from build123d import *

# Parameters (mm, degrees)
SKETCH2_W            = 100
SKETCH2_H            = 5.75
BOSS_EXTRUDE1_DEPTH  = 50
SKETCH4_R            = 11
CUT_EXTRUDE1_DEPTH   = 112.951161227
M3_CLEARANCE_HOLE2_D = 3.4
CUT_EXTRUDE3_DEPTH   = 5.75
FILLET1_R            = 25
FILLET2_R            = 10
M3_CLEARANCE_HOLE3_D = 3.4
SKETCH12_R           = 1
SKETCH12_W           = 24.5
SKETCH12_H           = 15
CUT_EXTRUDE4_DEPTH   = 5.75


with BuildPart() as part:
    # Sketch2 → Boss-Extrude1 (new body)
    with BuildSketch(Plane(origin=(0, 0, 0), x_dir=(1, 0, 0), z_dir=(0, 1, 0))):
        with Locations((-50, 2.875)):
            Rectangle(SKETCH2_W, SKETCH2_H)
    extrude(amount=BOSS_EXTRUDE1_DEPTH)

    # Sketch4 → Cut-Extrude1 (cut, through all)
    with BuildSketch(Plane.XY):
        with Locations((-25, 25)):
            Circle(SKETCH4_R)
    extrude(amount=-CUT_EXTRUDE1_DEPTH, mode=Mode.SUBTRACT)

    # M3 Clearance Hole2 (through all)
    with Locations(Plane.XY):
        with Locations((-35.606601718, 14.393398282), (-35.606601718, 35.606601718), (-14.393398282, 35.606601718), (-14.393398282, 14.393398282)):
            Hole(M3_CLEARANCE_HOLE2_D / 2)

    # Sketch9 → Cut-Extrude3 (cut)
    with BuildSketch(Plane.XY):
        with BuildLine():
            Line((-25, 50), (-100, 50))
            Line((-100, 50), (-100, 32.5))
            Line((-100, 32.5), (-48.848480035, 32.5))
            ThreePointArc((-48.848480035, 32.5), (-39.790199458, 45.155644371), (-25, 50))
        make_face()
        with BuildLine():
            Line((-25, 0), (-100, 0))
            Line((-100, 0), (-100, 17.5))
            Line((-100, 17.5), (-48.848480035, 17.5))
            ThreePointArc((-48.848480035, 17.5), (-39.790199458, 4.844355629), (-25, 0))
        make_face()
    extrude(amount=-CUT_EXTRUDE3_DEPTH, mode=Mode.SUBTRACT)

    # Fillet1
    fillet1_edges = [part.edges().sort_by_distance(p)[0] for p in [
        (0, 0, -2.875),
        (0, 50, -2.875),
    ]]
    fillet(fillet1_edges, radius=FILLET1_R - 0.0001)  # a hair under: the kernel refuses the full size

    # Fillet2
    fillet2_edges = [part.edges().sort_by_distance(p)[0] for p in [
        (-48.848480035, 32.5, -2.875),
        (-48.848480035, 17.5, -2.875),
    ]]
    fillet(fillet2_edges, radius=FILLET2_R)

    # M3 Clearance Hole3 (through all)
    with Locations(Plane.XY):
        with Locations((-94, 28.5), (-94, 21.5)):
            Hole(M3_CLEARANCE_HOLE3_D / 2)

    # Sketch12 → Cut-Extrude4 (cut)
    with BuildSketch(Plane.XY):
        with Locations((-70, 27.5)):
            Circle(SKETCH12_R)
        with Locations((-70, 22.5)):
            Circle(SKETCH12_R)
        with Locations((-87.75, 25)):
            Rectangle(SKETCH12_W, SKETCH12_H)
    extrude(amount=-CUT_EXTRUDE4_DEPTH, mode=Mode.SUBTRACT)


solid = part.part
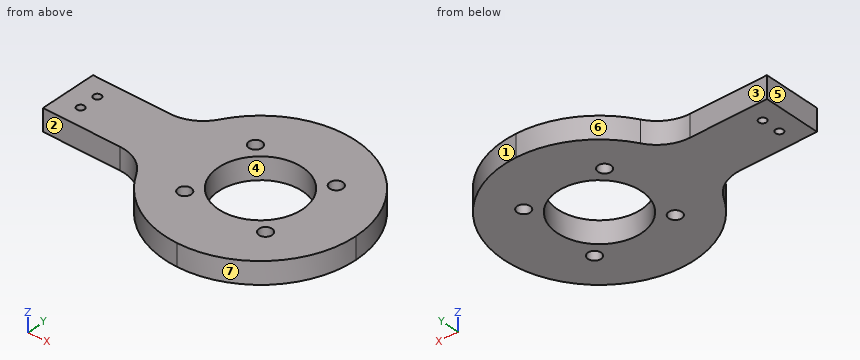
Work out the finished part from the listing and answer in its coordinate system (mm). Face numbers are marked on the shaded views. A direction names the side the tool comes from. Coordinates: 2 decimals unless noted, no trailing zeros. Loops run counter-clockwise (first coordinate to the right, second up) from the corner with the lowest first, then second, coordinate; pieces in that order, holes last. Notation, with made-up numbers: M 1,-10 L 23,-10 A29 cw 23,18 Z; hole C 44.5,62.5 d7. An arc over 180 degrees is marked long. Answer in a Markdown table with one row per item. Add a question column.
1. Consider L1, parallel to Y at x = -70, z = -2.25; L2, parallel to Y at x = -25, z = -4.2; L3, parallel to X at y = 37, z = -1.7. Determine where each line is inside the solid, lowest interval first.
2. The mould has two halves that part along Y. Classify the marked faces 4, 5, 6 and 7: pulls with the +Y half, pulls with the -Y half, needs draft (parallel to the pull), parting line crosses it, or undercut.
3. Find section A-A, the plane y = 22.5. Write down the section's boundary in (x, z), then the cut area to 3 significant figures.
4. Find section B-B, the plane x = -70. Write down the section's boundary in (y, z), then the cut area to 4 significant figures.
5. Find section C-C, the plane z = -4.5. State how many separate pieces and enclosed holes the cut face has, then the cut area to 3 significant figures.
6. Flat-ended cylindrical pins translate along their axes: P1, Ø2.5, axis at x = -35.61, y = 35.61, coming from the +Z side; P2, Ø2, axis at y = 13, z = -2.5, coming from the +X side; P3, Ø3, axis at y = 42, z = -3, coming from the -X side; P4, Ø1.5, axis at y = 41.5, z = -4.5, coming from the +X side. Find the tip coordinate at first contact, or state that the pin passes through.
7. A tool of negligible diameter and unlimited length cuts with its end or side. For the marked faces 1, 2 and 3, from which of +Z, -Z, +X, -X, +Y, -Y can it reach the whole face along a straight path? Write none if from no direction.
8. Find section D-D, the plane x = -21. Write down the section's boundary in (y, z).
Reported:
| question | item | result |
|---|---|---|
| 1 | L1 | y = 17.5 to 21.5, 23.5 to 26.5, 28.5 to 32.5 |
| 1 | L2 | y = 0 to 14, 36 to 50 |
| 1 | L3 | x = -46.96 to -36.58, -34.63 to -15.37, -13.42 to -3.07 |
| 2 | face 4 | undercut |
| 2 | face 5 | needs draft |
| 2 | face 6 | pulls with the +Y half |
| 2 | face 7 | pulls with the -Y half |
| 3 | outline | M -75.5,-5.75 L -71,-5.75 L -71,0 L -75.5,0 Z; M -69,-5.75 L -35.71,-5.75 L -35.71,0 L -69,0 Z; M -14.29,-5.75 L -0.13,-5.75 L -0.13,0 L -14.29,0 Z |
| 3 | area | 299 mm^2 |
| 4 | outline | M 17.5,-5.75 L 21.5,-5.75 L 21.5,0 L 17.5,0 Z; M 23.5,-5.75 L 26.5,-5.75 L 26.5,0 L 23.5,0 Z; M 28.5,-5.75 L 32.5,-5.75 L 32.5,0 L 28.5,0 Z |
| 4 | area | 63.25 mm^2 |
| 5 | separate pieces | 1 |
| 5 | enclosed holes | 7 |
| 5 | area | 1,940 mm^2 |
| 6 | P1 | passes through |
| 6 | P2 | stops at x = -2.55 |
| 6 | P3 | stops at x = -44.62 |
| 6 | P4 | stops at x = -5.59 |
| 7 | face 1 | +Z, -Z, +X, +Y |
| 7 | face 2 | +Z, -Z, -X, -Y |
| 7 | face 3 | +Z, -Z, -X, +Y |
| 8 | outline | M 0.32,-5.75 L 14.75,-5.75 L 14.75,0 L 0.32,0 Z; M 35.25,-5.75 L 49.68,-5.75 L 49.68,0 L 35.25,0 Z |
